from build123d import *

# Parameters (mm, degrees)
F1_DEPTH = 2.54
F0_W     = 1.27
F0_H     = 9.02178
F2_DEPTH = 27.94
F4_DEPTH = 25.4
F6_DEPTH = 38.1


with BuildPart() as f1:
    # F0 (on Top) → F1 (new body)
    with BuildSketch(Plane.XY):
        with BuildLine():
            Line((-382.154137, 163.215905), (-382.154137, 154.194125))
            Line((-382.154137, 154.194125), (-377.074137, 154.194125))
            Line((-377.074137, 154.194125), (-377.074137, 158.550225))
            ThreePointArc((-377.074137, 158.550225), (-379.068037, 160.544125), (-377.074137, 162.538025))
            Line((-377.074137, 162.538025), (-377.074137, 171.250225))
            ThreePointArc((-377.074137, 171.250225), (-379.068037, 173.244125), (-377.074137, 175.238025))
            Line((-377.074137, 175.238025), (-377.074137, 179.594125))
            Line((-377.074137, 179.594125), (-382.154137, 179.594125))
            Line((-382.154137, 179.594125), (-382.154137, 163.215905))
        make_face()
        with BuildLine():
            Line((-377.074137, 158.550225), (-377.074137, 154.194125))
            Line((-377.074137, 154.194125), (-371.994137, 154.194125))
            Line((-371.994137, 154.194125), (-371.994137, 179.594125))
            Line((-371.994137, 179.594125), (-377.074137, 179.594125))
            Line((-377.074137, 179.594125), (-377.074137, 175.238025))
            ThreePointArc((-377.074137, 175.238025), (-375.664237, 174.654025), (-375.080237, 173.244125))
            ThreePointArc((-375.080237, 173.244125), (-375.664237, 171.834224), (-377.074137, 171.250225))
            Line((-377.074137, 171.250225), (-377.074137, 162.538025))
            ThreePointArc((-377.074137, 162.538025), (-375.664237, 161.954025), (-375.080237, 160.544125))
            ThreePointArc((-375.080237, 160.544125), (-375.664237, 159.134224), (-377.074137, 158.550225))
        make_face()
    extrude(amount=F1_DEPTH)

    # F0 (on Top) → F2 (join)
    with BuildSketch(Plane.XY):
        Polygon((-383.424137, 182.134125), (-383.424137, 163.215905), (-382.154137, 163.215905), (-382.154137, 179.594125), (-377.074137, 179.594125), (-377.074137, 182.134125), align=None)
        Polygon((-371.994137, 179.594125), (-371.994137, 154.194125), (-370.724137, 154.194125), (-370.724137, 182.134125), (-377.074137, 182.134125), (-377.074137, 179.594125), align=None)
        with Locations((-382.789137, 158.705015)):
            Rectangle(F0_W, F0_H)
    extrude(amount=F2_DEPTH)

    # F3 (on face) → F4 (cut)
    with BuildSketch(Plane.XZ.offset(-179.594125)):
        with BuildLine():
            Line((-377.074137, 21.59), (-377.074137, 19.5961))
            ThreePointArc((-377.074137, 19.5961), (-375.664237, 20.1801), (-375.080237, 21.59))
            ThreePointArc((-375.080237, 21.59), (-375.664237, 22.9999), (-377.074137, 23.5839))
            Line((-377.074137, 23.5839), (-377.074137, 21.59))
        make_face()
        with BuildLine():
            ThreePointArc((-377.074137, 23.5839), (-379.068037, 21.59), (-377.074137, 19.5961))
            Line((-377.074137, 19.5961), (-377.074137, 21.59))
            Line((-377.074137, 21.59), (-377.074137, 23.5839))
        make_face()
        with BuildLine():
            ThreePointArc((-377.074137, 10.8839), (-379.068037, 8.89), (-377.074137, 6.8961))
            Line((-377.074137, 6.8961), (-377.074137, 8.89))
            Line((-377.074137, 8.89), (-377.074137, 10.8839))
        make_face()
        with BuildLine():
            Line((-377.074137, 8.89), (-377.074137, 6.8961))
            ThreePointArc((-377.074137, 6.8961), (-375.664237, 7.4801), (-375.080237, 8.89))
            ThreePointArc((-375.080237, 8.89), (-375.664237, 10.2999), (-377.074137, 10.8839))
            Line((-377.074137, 10.8839), (-377.074137, 8.89))
        make_face()
    extrude(amount=-F4_DEPTH, mode=Mode.SUBTRACT)

    # F5 (on face) → F6 (cut)
    with BuildSketch(Plane(origin=(-383.424137, 0, 0), x_dir=(0, -1, 0), z_dir=(-1, 0, 0))):
        Polygon((-159.582278, 5.388154), (-154.194125, 0), (-154.194125, 27.94), (-182.134125, 27.94), (-176.745971, 22.551846), (-176.745971, 5.388154), align=None)
    extrude(amount=-F6_DEPTH, mode=Mode.SUBTRACT)


solid = f1.part
Check sheet for the modelled part. Datum: model origin and axes. Units: mm. A direction names the side the tool comes from. Coordinates: 2 decimals unless noted, no trailing zeros. Write each loop counter-clockwise with the first axis right and the second up, starting at its lowest first coordinate (ties: lowest second). Pieces come first, ordered by that corner, then holes. Notation, with made-up numbers: M 43,71.25 L 90,71.25 A7 ccw 90,81.25 Z; hole C -36.5,86.5 d7. An arc over 180 degrees is marked long. Answer as CSV lines item,"result".
Q1. Mould release check, pull along X, two halves, no side actions. Record for faces 1 (the face through (-383.424, 175, 4)), 2 (the face through (-371, 176.746, 14)), 3 (the face through (-377, 179.594, 14)): released by +X, released by -X, zero draft, split by the parting line, or undercut.
Check result:
face 1,"released by -X"
face 2,"zero draft"
face 3,"undercut"
Q2. Cross-section at C-C (z = 20.5). Record the boundary of the cut face in (x, y), then the cut area to 3 significant figures.
Check result:
outline,"M -383.42,176.75 L -382.15,176.75 L -382.15,179.59 L -378.74,179.59 L -378.74,182.13 L -383.42,182.13 Z; M -375.4,179.59 L -371.99,179.59 L -371.99,176.75 L -370.72,176.75 L -370.72,182.13 L -375.4,182.13 Z"
area,"31.0 mm^2"
Q3. Set-up check for faces 4 (the face through (-377, 168, 2.54)), 5 (the face through (-377, 168, 0)), 6 (the face through (-383, 176.746, 14)): record each of +Z, -Z, +X, -X, +Y, -Y from which the full face is reachable in a straight line by a thin tool's end or side.
Check result:
face 4,"+Z, -Y"
face 5,"-Z, +X, -X, +Y, -Y"
face 6,"+Z, +X, -X, -Y"
Q4. Cross-section at D-D (x = -380). Record the boundary of the cut face in (y, z), then the cut area to 3 significant figures.
Check result:
outline,"M 154.19,0 L 182.13,0 L 182.13,27.94 L 179.59,25.4 L 179.59,2.54 L 156.73,2.54 Z"
area,"129 mm^2"
Q5. Cross-section at A-A (z = 13.5). Record the boundary of the cut face in (x, y), then the cut area to 3 significant figures.
Check result:
outline,"M -383.42,176.75 L -382.15,176.75 L -382.15,179.59 L -371.99,179.59 L -371.99,176.75 L -370.72,176.75 L -370.72,182.13 L -383.42,182.13 Z"
area,"39.5 mm^2"
Q6. Cross-section at B-B (x = -377.75). Record the boundary of the cut face in (y, z).
Check result:
outline,"M 154.19,0 L 158.67,0 L 158.67,2.54 L 156.73,2.54 Z; M 162.42,0 L 171.37,0 L 171.37,2.54 L 162.42,2.54 Z; M 175.12,0 L 182.13,0 L 182.13,7.01 L 179.59,7.01 L 179.59,2.54 L 175.12,2.54 Z; M 179.59,10.77 L 182.13,10.77 L 182.13,19.71 L 179.59,19.71 Z; M 179.59,23.47 L 182.13,23.47 L 182.13,27.94 L 179.59,25.4 Z"
Q7. Material ranges on probe 1 along X at (y, z) = (179, 7.25); probe 2 along Y at (x, z) = (-379.25, 8.5); probe 3 along Z at (x, y) = (-381.5, 158.75), recorded low to high. Write a range as from..to.
Check result:
probe 1,"-383.42..-382.15, -371.99..-370.72"
probe 2,"179.59..182.13"
probe 3,"0..2.54"
Q8. Go/stop test with flat-tipped pins: pin 1 (11.5 mm diameter, centred on y = 164, z = 14, fed in from +X); pin 2 (0.6 mm diameter, centred on x = -371, y = 171, fed in from +Z); pin 3 (0.6 mm diameter, centred on x = -371.5, z = 12.5, fed in from -Y); pin 4 (3 mm diameter, centred on x = -374, y = 171, fed in from +Z). Record where each tip stops, or that it passes through.
Check result:
pin 1,"through"
pin 2,"z = 5.39"
pin 3,"y = 176.75"
pin 4,"z = 2.54"
